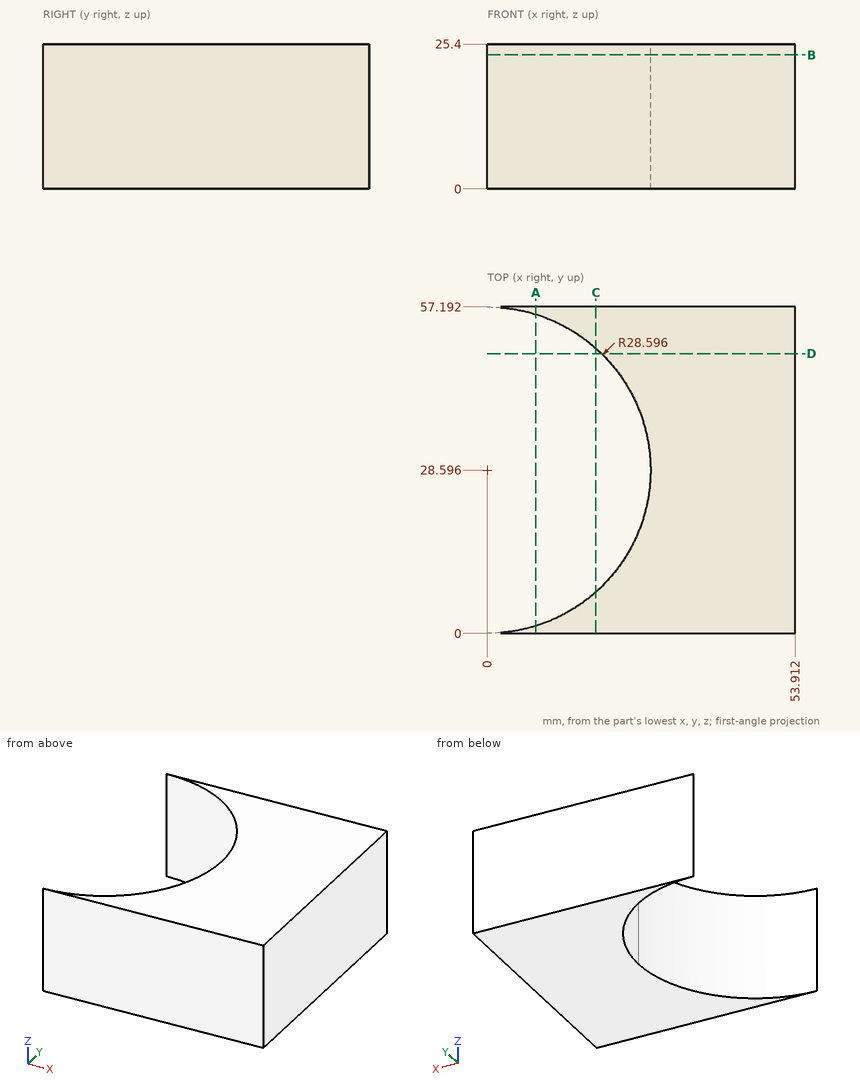
Check sheet for the drawn part. Datum: minimum x, y, z corner. Units: mm. Round coordinates to 2 decimals unless told otherwise and drop trailing zeros. Order: outer loops, then holes, each group sorted by start corner. A loop starts at its lowest first (then second) coordinate and runs counter-clockwise, first axis right, second up. Notation, with made-up numbers: M 55,32 L 68,32 A23 ccw 68,67 Z; hole C 5,-29 d3. An arc over 180 degrees is marked long. Write each question's results on one line, items separated by ' | '. Start each with the question number.
1. Cross-section at B-B on z = 23.5. Record the boundary of the cut face in (x, y).
2. Material ranges on L1, parallel to Y at x = 20, z = 19.75 (1 decimal); L2, parallel to Y at x = 23.5, z = 19 (1 decimal); L3, parallel to X at y = 53, z = 18 (1 decimal), recorded low to high. Write a range as from..to.
3. Cross-section at C-C on x = 19. Record the boundary of the cut face in (y, z) (1 decimal).
4. Cross-section at D-D on y = 49. Record the boundary of the cut face in (x, z) (1 decimal).
5. Go/stop test with flat-tipped pins: P1, Ø10, axis at y = 28.5, z = 16, coming from the -X side; P2, Ø4, axis at y = 48.5, z = 11, coming from the -X side (1 decimal); P3, Ø1.5, axis at y = 50, z = 18, coming from the -X side. Record where each tip stops, or that it passes through.
6. Cross-section at A-A on x = 8.5. Record the boundary of the cut face in (y, z).
Resolved:
1) outline: M 0,0 L 53.91,0 L 53.91,57.19 L 0,57.19 A28.6 cw 28.6,28.6 A28.6 cw Z
2) L1: 0..8.2, 49..57.2 | L2: 0..12.3, 44.9..57.2 | L3: 14.9..53.9
3) outline: M 0,0 L 7.2,0 L 7.2,25.4 L 0,25.4 Z; M 50,0 L 57.2,0 L 57.2,25.4 L 50,25.4 Z
4) outline: M 20,0 L 53.9,0 L 53.9,25.4 L 20,25.4 Z
5) P1: x = 28.14 | P2: x = 18.4 | P3: x = 18.08
6) outline: M 0,0 L 1.29,0 L 1.29,25.4 L 0,25.4 Z; M 55.9,0 L 57.19,0 L 57.19,25.4 L 55.9,25.4 Z
